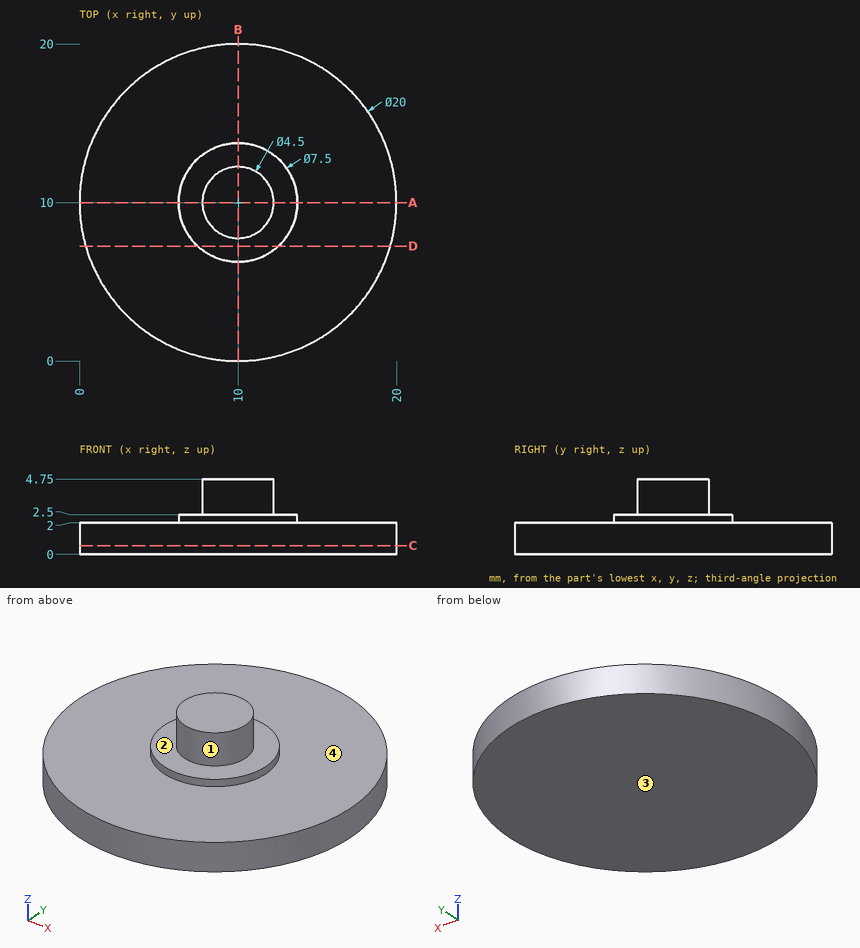
Check sheet for the drawn part. Datum: minimum x, y, z corner. Units: mm. A direction names the side the tool comes from. Give positions to 0.01 mm unless a question says otherwise; leave off trailing zeros. Write each loop counter-clockwise with the first axis right and the second up, starting at its lowest first coordinate (ties: lowest second). Pieces come first, ordered by that corner, then holes.
(1) Access from +Z, -Z, +X, -X, +Y, -Y to the whole of each face (thin tool, end or side, straight path). Record for the marked faces 3 and 4.
(2) Cross-section at A-A (y = 10). Enter the section's corners in (x, z), plus the area to 3 significant figures.
(3) Mould release check, pull along Y, two halves, no side actions. Record for the marked faces 1 and 2: +Y half, -Y half, draft (parallel to the pull), parting line (faces both ways), or undercut.
(4) Cross-section at D-D (y = 7.25). Enter the section's corners in (x, z), plus the area to 3 significant figures.
(5) Cross-section at C-C (z = 0.55). Enter the section's corners in (x, y), plus the area to 3 significant figures.
(6) Gauge pin test, flat ends, axial feed: pin 1 (1.5 mm diameter, centred on y = 16.5, z = 3.5, fed in from +X); pin 2 (1.5 mm diameter, centred on x = 3, y = 8.5, fed in from +Z). Record the tip position at first contact, or that the pin passes through.
(7) Material ranges on line 1 (Z direction, x = 18.25, y = 7); line 2 (X direction, y = 13, z = 2.4); line 3 (Z direction, x = 11.25, y = 7.25), recorded low to high.
Worked out:
1. face 3: -Z, +X, -X, +Y, -Y
1. face 4: +Z
2. outline: (0, 0) - (20, 0) - (20, 2) - (13.75, 2) - (13.75, 2.5) - (12.25, 2.5) - (12.25, 4.75) - (7.75, 4.75) - (7.75, 2.5) - (6.25, 2.5) - (6.25, 2) - (0, 2) - close
2. area: 53.9 mm2
3. face 1: parting line
3. face 2: draft
4. outline: (0.39, 0) - (19.61, 0) - (19.61, 2) - (12.55, 2) - (12.55, 2.5) - (7.45, 2.5) - (7.45, 2) - (0.39, 2) - close
4. area: 41.0 mm2
5. outline: circle Ø20 at (10, 10)
5. area: 314 mm2
6. pin 1: passes through
6. pin 2: stops at z = 2
7. line 1: z = 0 to 2
7. line 2: x = 7.75 to 12.25
7. line 3: z = 0 to 2.5
